from build123d import *

# Parameters (mm, degrees)
SKETCH1_R                = 15
BOSS_EXTRUDE1_DEPTH      = 20
SKETCH2_R                = 10.95
BOSS_EXTRUDE2_DEPTH      = 3.5
SKETCH4_R                = 3.05
CUT_EXTRUDE1_DEPTH       = 4.1
SKETCH5_R                = 1.5
CUT_EXTRUDE2_DEPTH       = 4
SKETCH7_R                = 10.95
SKETCH7_R_2              = 3
BOSS_EXTRUDE3_DEPTH      = 11
SKETCH9_R                = 1.5
CUT_EXTRUDE4_DEPTH       = 41.5
BOSS_EXTRUDE4_START      = 7
SKETCH12_R               = 18
SKETCH12_R_2             = 3.25
SKETCH12_R_3             = 3.05
BOSS_EXTRUDE4_DEPTH      = 7
CUT_EXTRUDE9_START       = -5
SKETCH13_R               = 1.5
CUT_EXTRUDE9_DEPTH       = 17
CIRPATTERN1_COUNT        = 3
CUT_EXTRUDE12_DEPTH      = 15
CUT_EXTRUDE12_DEPTH_BACK = 38.1079508
SKETCH15_R               = 13
SKETCH15_R_2             = 10.95
BOSS_EXTRUDE6_START      = 13
SKETCH17_R               = 13
BOSS_EXTRUDE6_DEPTH      = 20
SKETCH19_R               = 2.5
CUT_EXTRUDE13_DEPTH      = 38.107950728


with BuildPart() as part:
    # Sketch1 → Boss-Extrude1 (new body)
    with BuildSketch(Plane.XY):
        Circle(SKETCH1_R)
    extrude(amount=BOSS_EXTRUDE1_DEPTH)

    # Sketch2 → Boss-Extrude2 (add)
    with BuildSketch(Plane.XY.offset(20)):
        Circle(SKETCH2_R)
    extrude(amount=BOSS_EXTRUDE2_DEPTH)

    # Sketch4 → Cut-Extrude1 (cut)
    with BuildSketch(Plane(origin=(0, 0, 0), x_dir=(-1, 0, 0), z_dir=(0, 0, -1))):
        Circle(SKETCH4_R)
    extrude(amount=-CUT_EXTRUDE1_DEPTH, mode=Mode.SUBTRACT)

    # Sketch5 → Cut-Extrude2 (cut)
    with BuildSketch(Plane(origin=(0, 0, 4.1), x_dir=(-1, 0, 0), z_dir=(0, 0, -1))):
        Circle(SKETCH5_R)
    extrude(amount=-CUT_EXTRUDE2_DEPTH, mode=Mode.SUBTRACT)

    # Sketch7 → Boss-Extrude3 (add)
    with BuildSketch(Plane.XY.offset(23.5)):
        Circle(SKETCH7_R)
        Circle(SKETCH7_R_2, mode=Mode.SUBTRACT)
    extrude(amount=BOSS_EXTRUDE3_DEPTH)

    # Sketch9 → Cut-Extrude4 (cut, through all)
    with BuildSketch(Plane.XY.offset(34.5)):
        with Locations((7, 0)):
            Circle(SKETCH9_R)
        with Locations((-3.5, -6.062177826)):
            Circle(SKETCH9_R)
        with Locations((-3.5, 6.062177826)):
            Circle(SKETCH9_R)
    extrude(amount=-CUT_EXTRUDE4_DEPTH, mode=Mode.SUBTRACT)

    # Sketch12 → Boss-Extrude4 (add)
    with BuildSketch(Plane(origin=(0, 0, 0), x_dir=(-1, 0, 0), z_dir=(0, 0, -1)).offset(BOSS_EXTRUDE4_START)):
        Circle(SKETCH12_R)
        with Locations((3.5, 6.062177826)):
            Circle(SKETCH12_R_2, mode=Mode.SUBTRACT)
        with Locations((3.5, -6.062177826)):
            Circle(SKETCH12_R_2, mode=Mode.SUBTRACT)
        with Locations((-7, 0)):
            Circle(SKETCH12_R_2, mode=Mode.SUBTRACT)
        Circle(SKETCH12_R_3, mode=Mode.SUBTRACT)
    extrude(amount=-BOSS_EXTRUDE4_DEPTH)

    # Sketch13 → Cut-Extrude9 (cut)
    with BuildSketch(Plane(origin=(0, 0, 0), x_dir=(0, 0, -1), z_dir=(1, 0, 0)).offset(CUT_EXTRUDE9_START)):
        with Locations((2, 0)):
            Circle(SKETCH13_R)
    cut_extrude9 = extrude(amount=-CUT_EXTRUDE9_DEPTH, mode=Mode.SUBTRACT)

    # CirPattern1: Cut-Extrude9 ×3 about axis
    cirpattern1_axis = Axis((0, 0, 0), (0, 0, 1))
    for i in range(1, CIRPATTERN1_COUNT):
        add(cut_extrude9.rotate(cirpattern1_axis, i * 360 / CIRPATTERN1_COUNT), mode=Mode.SUBTRACT)

    # Sketch15 → Cut-Extrude12 (cut, two sides: drawn at the far end of the back side and taken through both)
    # profile 1 of 2: a face of its own
    with BuildSketch(Plane.XY.offset(20).offset(-CUT_EXTRUDE12_DEPTH_BACK)):
        Circle(SKETCH15_R)
        Circle(SKETCH15_R_2, mode=Mode.SUBTRACT)
    # profile 2 of 2: a face of its own
    with BuildSketch(Plane.XY.offset(20).offset(-CUT_EXTRUDE12_DEPTH_BACK)):
        Circle(SKETCH15_R_2)
    extrude(amount=CUT_EXTRUDE12_DEPTH + CUT_EXTRUDE12_DEPTH_BACK, mode=Mode.SUBTRACT)

    # Sketch17 → Boss-Extrude6 (add)
    with BuildSketch(Plane.XY.offset(BOSS_EXTRUDE6_START)):
        Circle(SKETCH17_R)
    extrude(amount=-BOSS_EXTRUDE6_DEPTH)

    # Sketch19 → Cut-Extrude13 (cut, through all)
    with BuildSketch(Plane(origin=(0, 0, -7), x_dir=(-1, 0, 0), z_dir=(0, 0, -1))):
        with Locations((7.66, 0)):
            Circle(SKETCH19_R)
        with Locations((-3.83, -6.633754593)):
            Circle(SKETCH19_R)
        with Locations((-3.83, 6.633754593)):
            Circle(SKETCH19_R)
    extrude(amount=-CUT_EXTRUDE13_DEPTH, mode=Mode.SUBTRACT)


solid = part.part
CAD build for the part. Positions are in the model's coordinates, mm. A direction names the side the tool comes from. Round coordinates to 2 decimals unless told otherwise and drop trailing zeros. Write each loop counter-clockwise with the first axis right and the second up, starting at its lowest first coordinate (ties: lowest second). Pieces come first, ordered by that corner, then holes. Notation, with made-up numbers: (64.5, 25.25) -> (77.5, 25.25) arc R16 cw to (77.5, 32.25) -> close; hole circle Ø2 at (56, -24). An arc over 180 degrees is marked (long way). Answer as a JSON object with one key per item and string values.
(1) Band-saw the part on A-A, the plane x = 0. List the corners of the cut face in (y, z).
Reported:
{"outline": "(-18, -7) -> (18, -7) -> (18, 0) -> (15, 0) -> (15, 20) -> (13, 20) -> (13, 13) -> (-13, 13) -> (-13, 20) -> (-15, 20) -> (-15, 0) -> (-18, 0) -> close"}
(2) Band-saw the part on B-B, the plane z = -2. List the corners of the cut face in (x, y).
Reported:
{"outline": "(-17.94, -1.5) arc R18 ccw to (7.67, -16.28) -> (5.16, -11.93) arc R13 ccw to (7.76, -10.43) -> (10.27, -14.78) arc R18 ccw to (10.27, 14.78) -> (7.76, 10.43) arc R13 ccw to (5.16, 11.93) -> (7.67, 16.28) arc R18 ccw to (-17.94, 1.5) -> (-12.91, 1.5) arc R13 ccw to (-12.91, -1.5) -> close; hole circle Ø5 at (-7.66, 0); hole circle Ø5 at (3.83, -6.63); hole circle Ø5 at (3.83, 6.63)"}
(3) Probe probe 1 along Y at (x, z) = (-7.66, -1.5); probe 2 along Z at (x, y) = (-14, 0); probe 3 along Z at (x, y) = (-5, -10). List the from-to ranges inside material, lowest first. Write a range as [from, to].
Reported:
{"probe 1": "y = [-16.29, -2.5], [2.5, 16.29]", "probe 2": "z = [-7, -3.5], [-0.5, 20]", "probe 3": "z = [-7, 13]"}
(4) Band-saw the part on C-C, the plane y = 0.5. List the corners of the cut face in (x, z).
Reported:
{"outline": "(-17.99, -7) -> (-10.11, -7) -> (-10.11, 13) -> (-12.99, 13) -> (-12.99, 20) -> (-14.99, 20) -> (-14.99, 0) -> (-17.99, 0) -> (-17.99, -0.59) -> (-12.99, -0.59) -> (-12.99, -3.41) -> (-17.99, -3.41) -> close; (-5.21, -7) -> (17.99, -7) -> (17.99, 0) -> (14.99, 0) -> (14.99, 20) -> (12.99, 20) -> (12.99, 13) -> (-5.21, 13) -> close"}
(5) Pin check, flat tips, straight feed: P1, Ø4, axis at y = 2, z = 4.5, coming from the -X side; P2, Ø8, axis at y = -13, z = -1.5, coming from the +X side; P3, Ø5, axis at x = 3, z = 14.5, coming from the -Y side. Stop position of each tip, or through.
Reported:
{"P1": "stops at x = -15", "P2": "stops at x = 15.59", "P3": "stops at y = -14.99"}
(6) Band-saw the part on D-D, the plane x = 3.83. List the corners of the cut face in (y, z), then the cut area to 3 significant figures.
Reported:
{"outline": "(-17.59, -7) -> (-9.13, -7) -> (-9.13, 13) -> (-12.42, 13) -> (-12.42, 20) -> (-14.5, 20) -> (-14.5, 0) -> (-17.59, 0) -> close; (-4.13, -7) -> (4.13, -7) -> (4.13, 13) -> (-4.13, 13) -> close; (9.13, -7) -> (17.59, -7) -> (17.59, 0) -> (14.5, 0) -> (14.5, 20) -> (12.42, 20) -> (12.42, 13) -> (9.13, 13) -> close", "area": "452 mm^2"}
(7) Which spindle directions (+Z, -Z, +X, -X, +Y, -Y) get a long thin tool onto all of the face, cutting with end or side? Do faces 1 (the face through (-14.985, 0.66, 9.86)), 2 (the face through (-15.42, 0.07, -0.5)), 3 (the face through (-0.1, 13.4, 20)), 4 (the face through (2.343, 17.847, -3.549)), 5 (the face through (6.48, -11.27, -1.97)). Say none if no direction does.
Reported:
{"face 1": "+Z", "face 2": "-X", "face 3": "+Z, +X, -X, +Y, -Y", "face 4": "+Z, -Z", "face 5": "none"}
(8) Two-plate mould, pull along Z, no slides. Class faces 6 (the face through (6.519, 11.247, -1.973)), 7 (the face through (-5.162, 0.11, 2.86)), 8 (the face through (8.5, -12.9, -0.81)), 9 (the face through (0, 0, -7)): +Z half, -Z half, draft (parallel to the pull), parting line (faces both ways), or undercut.
Reported:
{"face 6": "undercut", "face 7": "draft", "face 8": "undercut", "face 9": "-Z half"}
